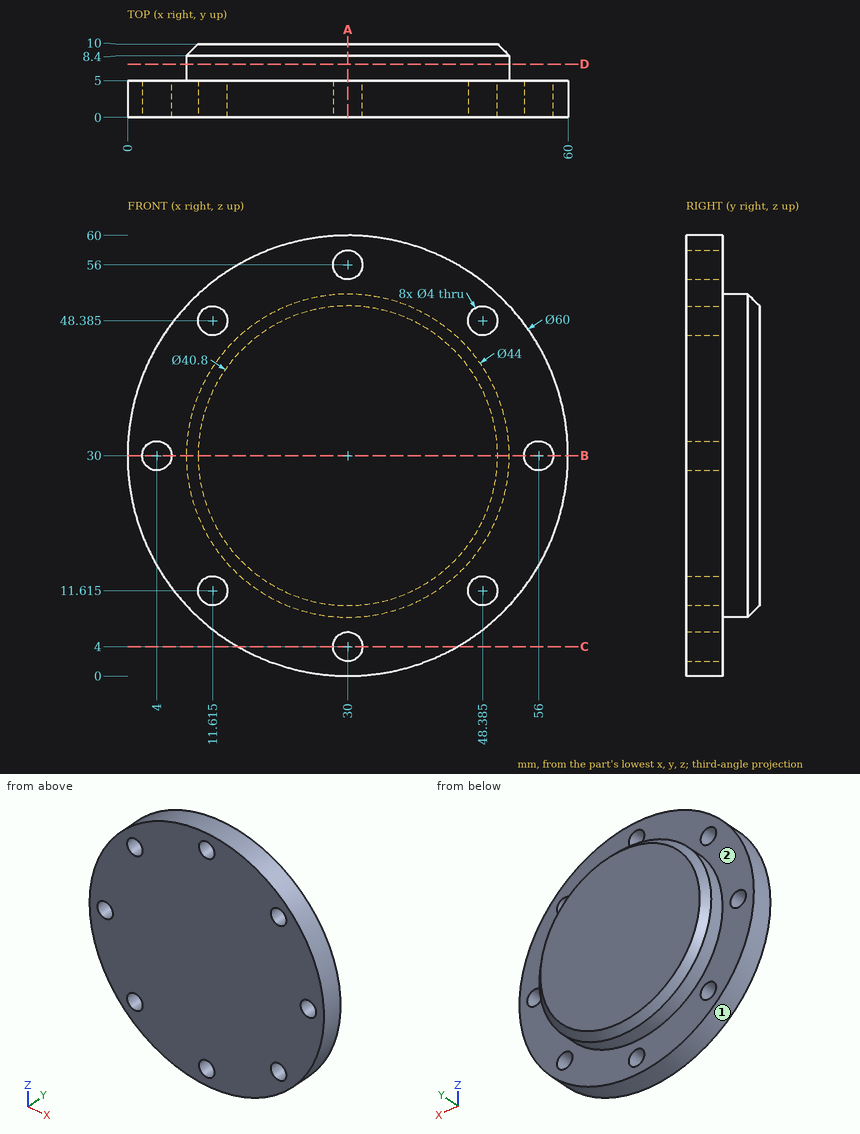
Geometry check sheet. Reference: drawing and pictorial views, mm from the part's lowest x, y, z. A direction names the side the tool comes from. Coordinates: 2 decimals unless noted, no trailing zeros. Order: outer loops, then holes, each group sorted by start corner. A loop starts at its lowest first (then second) coordinate and runs counter-clockwise, first axis right, second up.
Item 1: Section check C-C (z = 4). Enter the section's corners in (x, y).
Item 2: Depth check by flat-ended pin: pin 1 (6 mm diameter, centred on y = 3, z = 46.5, fed in from +X); pin 2 (6 mm diameter, centred on y = 4, z = 34, fed in from +X); pin 3 (4.5 mm diameter, centred on x = 48.38, z = 11.62, fed in from +Y). Enter the tip coordinate at first touch or a pass-through.
Item 3: Tool access check on the marked faces 1 and 2. Record the directions out of +Z, -Z, +X, -X, +Y, -Y that give a thin tool (end or side, any length) a straight path to the whole face; none if there is none.
Item 4: Section check B-B (z = 30). Enter the section's corners in (x, y).
Item 5: Scan lines: line 1 along X through (y, z) = (1.5, 28.5); line 2 along Z through (x, y) = (49.5, 4.75) (1 decimal); line 3 along X through (y, z) = (1, 8) (1 decimal). Record each from-to range of solid material in increasing order.
Item 6: Section check A-A (x = 30). Enter the section's corners in (y, z).
Item 7: Section check D-D (y = 7.25). Enter the section's corners in (x, z), plus the area to 3 significant figures.
Check sheet entries:
1. outline: (15.03, 0) - (28, 0) - (28, 5) - (15.03, 5) - close; (32, 0) - (44.97, 0) - (44.97, 5) - (32, 5) - close
2. pin 1: stops at x = 56.79
2. pin 2: stops at x = 59.98
2. pin 3: stops at y = 5
3. face 1: +Y, -Y
3. face 2: +Y
4. outline: (0, 0) - (2, 0) - (2, 5) - (0, 5) - close; (6, 0) - (54, 0) - (54, 5) - (52, 5) - (52, 8.4) - (50.4, 10) - (9.6, 10) - (8, 8.4) - (8, 5) - (6, 5) - close; (58, 0) - (60, 0) - (60, 5) - (58, 5) - close
5. line 1: x = 0.04 to 2.68, 5.32 to 54.68, 57.32 to 59.96
5. line 2: z = 7.2 to 10, 13.3 to 46.7, 50 to 52.8
5. line 3: x = 9.6 to 50.4
6. outline: (0, 0) - (5, 0) - (5, 2) - (0, 2) - close; (0, 6) - (5, 6) - (5, 8) - (8.4, 8) - (10, 9.6) - (10, 50.4) - (8.4, 52) - (5, 52) - (5, 54) - (0, 54) - close; (0, 58) - (5, 58) - (5, 60) - (0, 60) - close
7. outline: circle Ø44 at (30, 30)
7. area: 1,520 mm2
